Geometry: final body of the model. Coordinates: model frame, mm. Face numbers are marked on the shaded views. A direction names the side the tool comes from. Give positions to 0.01 mm unless a question says otherwise; leave off trailing zeros. Loops run counter-clockwise (first coordinate to the right, second up) from the corner with the lowest first, then second, coordinate; pieces in that order, holes last. Notation, with made-up numbers: M 33.5,27 L 83.5,27 A21 cw 83.5,31 Z; hole C -10.5,13 d4. An arc over 180 degrees is marked long. Put each result on its own line as item: value.
```python
from build123d import *

# Parameters (mm, degrees)
F1_DEPTH = 76.2
F2_R     = 21.590363
F3_DEPTH = 63.501
F4_W     = 9.904528
F4_H     = 58.43965
F5_DEPTH = 50.8
F7_DEPTH = 25.4


with BuildPart() as f1:
    # F0 (on Front) → F1 (new body)
    with BuildSketch(Plane.XZ):
        Polygon((-46.429671, -13.227126), (-46.429671, -38.627126), (42.470329, -38.627126), (42.470329, -13.227126), (17.070329, -13.227126), (17.070329, 50.272874), (42.470329, 50.272874), (42.470329, 75.672874), (-46.429671, 75.672874), (-46.429671, 50.272874), (-21.029671, 50.272874), (-21.029671, -13.227126), align=None)
    extrude(amount=F1_DEPTH)

    # F2 (on face) → F3 (cut, through all)
    with BuildSketch(Plane.YZ.offset(17.070329)):
        with Locations((-38.1, 18.522874)):
            Circle(F2_R)
    extrude(amount=-F3_DEPTH, mode=Mode.SUBTRACT)

    # F4 (on face) → F5 (join)
    with BuildSketch(Plane.XY.offset(75.672874)):
        with Locations((0, -38.1)):
            Rectangle(F4_W, F4_H)
    extrude(amount=F5_DEPTH)

    # F6 (on face) → F7 (join)
    with BuildSketch(Plane.YZ.offset(4.952264)):
        Polygon((-19.896209, 95.37485), (-27.760912, 117.595732), (-51.324553, 116.982586), (-58.022983, 94.382759), (-38.599198, 81.028443), align=None)
    extrude(amount=F7_DEPTH)


solid = f1.part
```
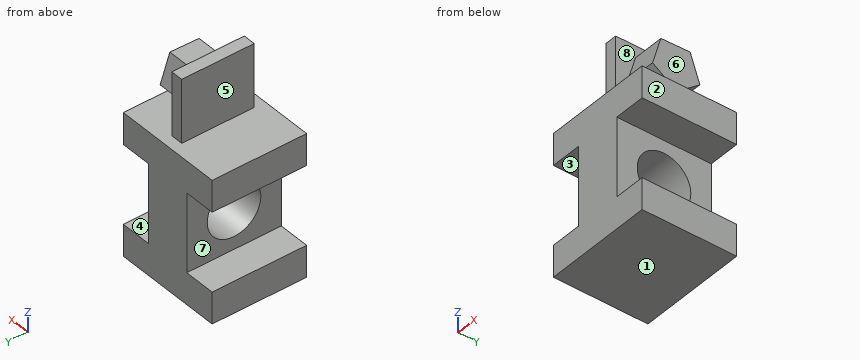
Item 1: Mould query, pull axis Z, two halves, no side actions, for the marked faces 1, 2 and 3. Classes: pulls with the +Z half, pulls with the -Z half, needs draft (parallel to the pull), parting line crosses it, or undercut.
Output values:
face 1: pulls with the -Z half
face 2: needs draft
face 3: undercut
Item 2: Section B-B on x = 34.5. Output: boundary loops of the cut face in (y, z), then the cut area to 3 significant figures.
Output values:
outline: M -76.2,-38.63 L 0,-38.63 L 0,-13.23 L -76.2,-13.23 Z; M -76.2,50.27 L 0,50.27 L 0,75.67 L -76.2,75.67 Z
area: 3,870 mm²
Item 3: Section C-C on z = 36.5. Output: boundary loops of the cut face in (x, y).
Output values:
outline: M -21.03,-76.2 L 17.07,-76.2 L 17.07,-50.06 L -21.03,-50.06 Z; M -21.03,-26.14 L 17.07,-26.14 L 17.07,0 L -21.03,0 Z
Item 4: Section D-D on x = 9.5. Output: boundary loops of the cut face in (y, z), then the cut area to 3 significant figures.
Output values:
outline: M -76.2,-38.63 L 0,-38.63 L 0,75.67 L -76.2,75.67 Z; M -58.02,94.38 L -38.6,81.03 L -19.9,95.37 L -27.76,117.6 L -51.32,116.98 Z; hole C -38.1,18.52 d43.18
area: 8,200 mm²
Item 5: Line query: probe 1 along Z at (x, y) = (-3, -38); probe 2 along Z at (x, y) = (25, -5.5); probe 3 along Z at (x, y) = (5, -38). Output: solid intervals per line, ascending. Write a range as [from, to].
Output values:
probe 1: [-38.63, -3.07], [40.11, 126.47]
probe 2: [-38.63, -13.23], [50.27, 75.67]
probe 3: [-38.63, -3.07], [40.11, 75.67], [81.49, 117.33]
Item 6: Set-up query: the marked faces 4, 5, 6, 7 and 8. Return all of +Z, -Z, +X, -X, +Y, -Y with unobstructed straight access to the full face (end or side cutting, diameter ignored); none if empty.
Output values:
face 4: +X, +Y, -Y
face 5: +Z, -X, +Y, -Y
face 6: +Z, +X, +Y, -Y
face 7: -X, +Y, -Y
face 8: +X
Item 7: Pin query (flat end, axial travel): pin 1 Ø12.5 at (x, y) = (26.5, -46.5) entering from +Z; pin 2 Ø10 at (y, z) = (-20, -4.5) entering from +X; pin 3 Ø1 at (x, y) = (-12, -55) entering from +Z. Return the tip coordinate at first contact, or that it passes through.
Output values:
pin 1: z = 117.27
pin 2: x = 17.07
pin 3: z = 75.67
Item 8: Section A-A on x = 19. Output: boundary loops of the cut face in (y, z), then the cut area to 3 significant figures.
Output values:
outline: M -76.2,-38.63 L 0,-38.63 L 0,-13.23 L -76.2,-13.23 Z; M -76.2,50.27 L 0,50.27 L 0,75.67 L -76.2,75.67 Z; M -58.02,94.38 L -38.6,81.03 L -19.9,95.37 L -27.76,117.6 L -51.32,116.98 Z
area: 4,830 mm²
